Verification items for this drawing (mm, ordinates from the low corner). A direction names the side the tool comes from. Give positions to 0.01 mm unless a question says otherwise; leave off trailing zeros. Loops run counter-clockwise (first coordinate to the right, second up) from the corner with the lowest first, then second, coordinate; pieces in that order, holes last. Notation, with made-up numbers: M 38,64.25 L 58,64.25 A21 ccw 58,99.25 Z; hole C 75,23.25 d10. An arc over 180 degrees is marked long. Answer in a Markdown table with one row per item.
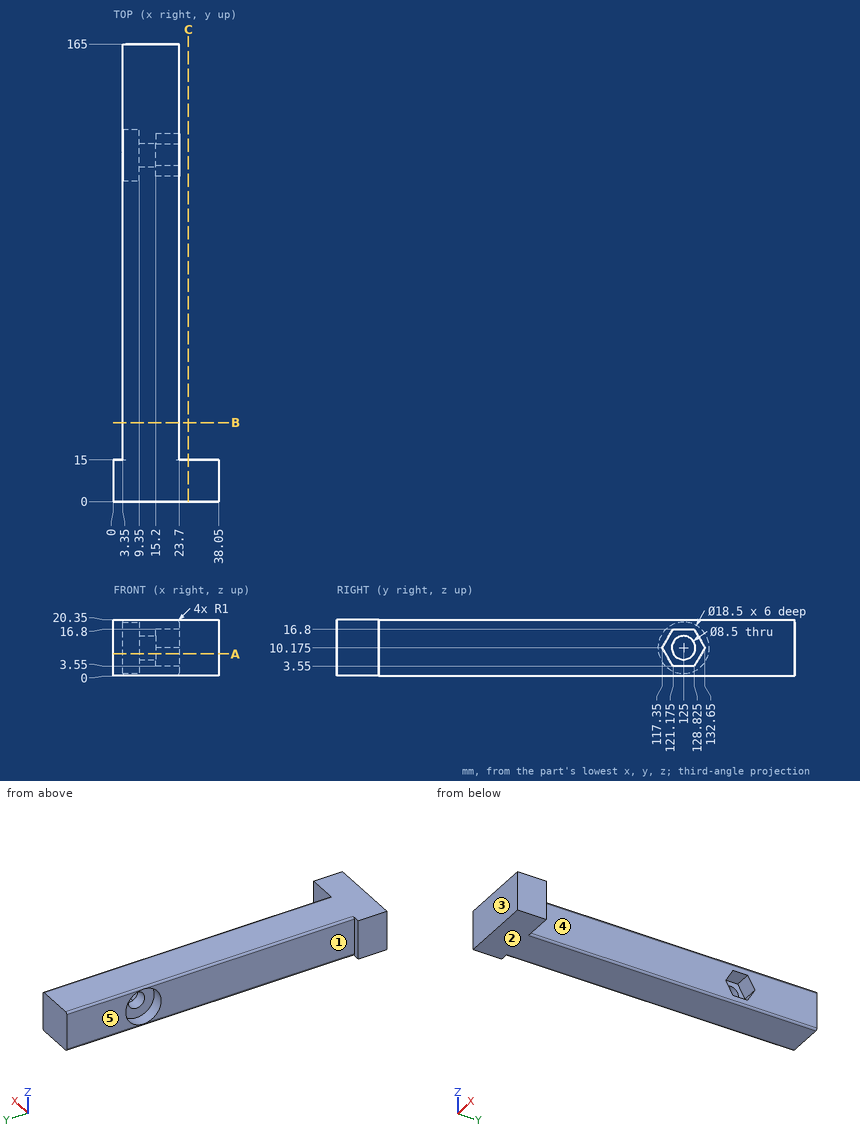
Item 1: Release check for a two-part mould opening along X. For the marked faces 3, 4 and 5 record: released by +X, released by -X, zero draft, split by the parting line, or undercut.
Reported:
| item | result |
|---|---|
| face 3 | zero draft |
| face 4 | released by +X |
| face 5 | released by -X |
Item 2: Tool access check on the marked faces 1 and 2. Record the directions out of +Z, -Z, +X, -X, +Y, -Y that give a thin tool (end or side, any length) a straight path to the whole face; none if there is none.
Reported:
| item | result |
|---|---|
| face 1 | +Z, -Z, -X, +Y |
| face 2 | -Z, +X, -X, +Y, -Y |
Item 3: Sectioned sample at C-C (x = 27). Record the cut outline in (y, z).
Reported:
| item | result |
|---|---|
| outline | M 0,0 L 15,0 L 15,20.35 L 0,20.35 Z |
Item 4: Sectioned sample at A-A (z = 8). Record the cut outline in (x, y), and give its area (3 significant figures).
Reported:
| item | result |
|---|---|
| outline | M 0,0 L 38.05,0 L 38.05,15 L 23.7,15 L 23.7,118.61 L 15.2,118.61 L 15.2,121.35 L 9.35,121.35 L 9.35,116.01 L 3.35,116.01 L 3.35,15 L 0,15 Z; M 3.35,133.99 L 9.35,133.99 L 9.35,128.65 L 15.2,128.65 L 15.2,131.39 L 23.7,131.39 L 23.7,165 L 3.35,165 Z |
| area | 3,360 mm^2 |
Item 5: Go/stop test with flat-tipped pins: pin 1 (5 mm diameter, centred on y = 125, z = 10.175, fed in from -X); pin 2 (6 mm diameter, centred on x = 9.5, z = 3.5, fed in from -Y); pin 3 (5 mm diameter, centred on y = 88, z = 15.5, fed in from -X); pin 4 (4.5 mm diameter, centred on x = 29, z = 9.5, fed in from +Y). Record where each tip stops, or that it passes through.
Reported:
| item | result |
|---|---|
| pin 1 | passes through |
| pin 2 | stops at y = 0 |
| pin 3 | stops at x = 3.35 |
| pin 4 | stops at y = 15 |
Item 6: Sectioned sample at B-B (y = 28.5). Record the cut outline in (x, z).
Reported:
| item | result |
|---|---|
| outline | M 3.35,1 A1 ccw 4.35,0 L 22.7,0 A1 ccw 23.7,1 L 23.7,19.35 A1 ccw 22.7,20.35 L 4.35,20.35 A1 ccw 3.35,19.35 Z |
Item 7: Scan lines: L1, parallel to Z at x = 13.55, y = 125 (3 decimals); L2, parallel to Z at x = 6, y = 125 (3 decimals); L3, parallel to X at y = 22.5, z = 7.5. Record each from-to range of solid material in increasing order. Write a range as [from, to].
Reported:
| item | result |
|---|---|
| L1 | z = [0, 5.925], [14.425, 20.35] |
| L2 | z = [0, 0.925], [19.425, 20.35] |
| L3 | x = [3.35, 23.7] |
